```python
from build123d import *

# Parameters (mm, degrees)
LINEAR_AUSTRAGEN_D_NN1_DEPTH    = 50
SKIZZE2_R                       = 11.05
SKIZZE2_R_2                     = 1.75
SCHNITT_LINEAR_AUSTRAGEN1_DEPTH = 2.5
AUFSATZ_LINEAR_AUSTRAGEN1_DEPTH = 1.5
SCHNITT_LINEAR_AUSTRAGEN2_DEPTH = 2.5
FASE1_SIZE                      = 5


with BuildPart() as part:
    # Skizze1 → Linear-Austragen-Dünn1 (new body)
    with BuildSketch(Plane(origin=(0, 0, 0), x_dir=(0, 0, -1), z_dir=(1, 0, 0))):
        with BuildLine():
            Line((53.5, 0), (2, 0))
            ThreePointArc((2, 0), (0.585786438, 0.585786438), (0, 2))
            Line((0, 2), (0, 50.5))
            Line((0, 50.5), (1.5, 50.5))
            Line((1.5, 50.5), (1.5, 2))
            ThreePointArc((1.5, 2), (1.646446609, 1.646446609), (2, 1.5))
            Line((2, 1.5), (53.5, 1.5))
            Line((53.5, 1.5), (53.5, 0))
        make_face()
    extrude(amount=LINEAR_AUSTRAGEN_D_NN1_DEPTH)

    # Skizze2 → Schnitt-Linear austragen1 (cut, through all)
    with BuildSketch(Plane(origin=(0, 0, -1.5), x_dir=(-1, 0, 0), z_dir=(0, 0, -1))):
        with Locations((-25, 29.5)):
            Circle(SKIZZE2_R)
        with Locations((-40.5, 45)):
            Circle(SKIZZE2_R_2)
        with Locations((-9.5, 45)):
            Circle(SKIZZE2_R_2)
        with Locations((-9.5, 14)):
            Circle(SKIZZE2_R_2)
        with Locations((-40.5, 14)):
            Circle(SKIZZE2_R_2)
    extrude(amount=-SCHNITT_LINEAR_AUSTRAGEN1_DEPTH, mode=Mode.SUBTRACT)

    # Skizze3 → Aufsatz-Linear austragen1 (add)
    with BuildSketch(Plane(origin=(50, 0, 0), x_dir=(0, 0, -1), z_dir=(1, 0, 0))):
        Polygon((1.5, 21.5), (14.5, 1.5), (3.5, 1.5), (1.5, 4.576923077), align=None)
    aufsatz_linear_austragen1 = extrude(amount=-AUFSATZ_LINEAR_AUSTRAGEN1_DEPTH)

    # Spiegeln1: Aufsatz-Linear austragen1 across plane
    add(aufsatz_linear_austragen1.mirror(Plane(origin=(25, 0, 0), x_dir=(0, 0, 1), z_dir=(1, 0, 0))))

    # Skizze4 → Schnitt-Linear austragen2 (cut, through all)
    with BuildSketch(Plane(origin=(0, 1.5, 0), x_dir=(1, 0, 0), z_dir=(0, 1, 0))):
        with BuildLine():
            Line((7.9, 13.706666488), (7.9, 41.293333512))
            ThreePointArc((7.9, 41.293333512), (10, 43.393333512), (12.1, 41.293333512))
            Line((12.1, 41.293333512), (12.1, 13.706666488))
            ThreePointArc((12.1, 13.706666488), (10, 11.606666488), (7.9, 13.706666488))
        make_face()
        with BuildLine():
            Line((42.1, 13.706666488), (42.1, 41.293333512))
            ThreePointArc((42.1, 41.293333512), (40, 43.393333512), (37.9, 41.293333512))
            Line((37.9, 41.293333512), (37.9, 13.706666488))
            ThreePointArc((37.9, 13.706666488), (40, 11.606666488), (42.1, 13.706666488))
        make_face()
    extrude(amount=-SCHNITT_LINEAR_AUSTRAGEN2_DEPTH, mode=Mode.SUBTRACT)

    # Fase1
    fase1_edges = [part.edges().sort_by_distance(p)[0] for p in [
        (50, 50.5, -0.75),
        (50, 0.75, -53.5),
        (0, 50.5, -0.75),
        (0, 0.75, -53.5),
    ]]
    chamfer(fase1_edges, length=FASE1_SIZE)


solid = part.part
```
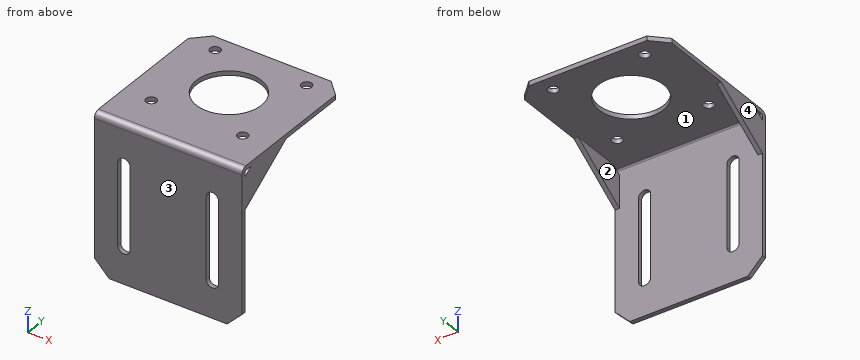
Verification items for the finished model (mm, model axes). Face numbers are marked on the shaded views. Round coordinates to 2 decimals unless told otherwise and drop trailing zeros. Write each loop counter-clockwise with the first axis right and the second up, starting at its lowest first coordinate (ties: lowest second). Pieces come first, ordered by that corner, then holes.
1. Draft check along X on the marked faces 1, 2, 3 and 4. Enter one of: +X half, -X half, draft (parallel to the pull), parting line (faces both ways), or undercut.
2. Section check A-A on x = 25. Enter the section's corners in (y, z), plus the area to 3 significant figures.
3. Section check B-B on z = -39.5. Enter the section's corners in (x, y), plus the area to 3 significant figures.
4. Gauge pin test, flat ends, axial feed: P1, Ø5, axis at x = 19.5, z = -34, coming from the +Y side; P2, Ø1, axis at x = 15, y = 8.5, coming from the -Z side. Record the tip position at first contact, or that the pin passes through.
5. Section check D-D on x = 46.5. Enter the section's corners in (y, z).
6. Section check C-C on y = 29.5. Enter the section's corners in (x, z).
7. Scan lines: L1, parallel to Z at x = 36, y = 25; L2, parallel to Y at x = 25, z = -16.5; L3, parallel to Y at x = 40.5, z = -0.75. Record each from-to range of solid material in increasing order.
Answer:
1. face 1: undercut
1. face 2: undercut
1. face 3: draft
1. face 4: -X half
2. outline: (0, -53.5) - (1.5, -53.5) - (1.5, -2) arc R0.5 cw to (2, -1.5) - (18.45, -1.5) - (18.45, 0) - (2, 0) arc R2 ccw to (0, -2) - close; (40.55, -1.5) - (50.5, -1.5) - (50.5, 0) - (40.55, 0) - close
2. area: 120 mm2
3. outline: (0, 0) - (7.9, 0) - (7.9, 1.5) - (0, 1.5) - close; (12.1, 0) - (37.9, 0) - (37.9, 1.5) - (12.1, 1.5) - close; (42.1, 0) - (50, 0) - (50, 1.5) - (42.1, 1.5) - close
3. area: 62.4 mm2
4. P1: stops at y = 1.5
4. P2: stops at z = -1.5
5. outline: (0, -52) - (1.5, -52) - (1.5, -2) arc R0.5 cw to (2, -1.5) - (49, -1.5) - (49, 0) - (2, 0) arc R2 ccw to (0, -2) - close
6. outline: (0, -1.5) - (13.95, -1.5) - (13.95, 0) - (0, 0) - close; (36.05, -1.5) - (50, -1.5) - (50, 0) - (36.05, 0) - close
7. L1: z = -1.5 to 0
7. L2: y = 0 to 1.5
7. L3: y = 0.44 to 12.25, 15.75 to 43.25, 46.75 to 50.5
